The model under review builds one solid part; all positions refer to its coordinate system, in mm. Face numbers are marked on the shaded views. A direction names the side the tool comes from. Coordinates: 2 decimals unless noted, no trailing zeros. Order: outer loops, then holes, each group sorted by start corner. A loop starts at its lowest first (then second) coordinate and runs counter-clockwise, first axis right, second up.
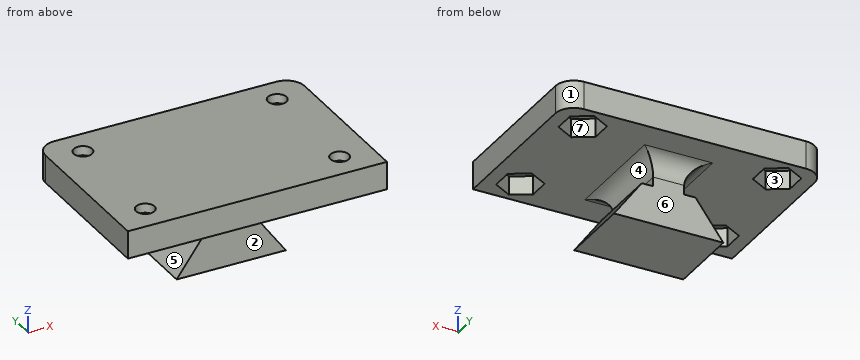
```python
from build123d import *

# Parameters (mm, degrees)
DOVETAIL_DEPTH     = 8
SKETCH2_W          = 3.35034124
SKETCH2_H          = 8
STEM_DEPTH         = 3
SKETCH3_W          = 28
SKETCH3_H          = 18.5
CAMERA_PLATE_DEPTH = 3
FILLET1_R          = 2
SKETCH4_R          = 1
SCREW_HOLES_DEPTH  = 3
NUT_HOLES_DEPTH    = 2
FILLET2_R          = 2


with BuildPart() as part:
    # Sketch1 → Dovetail (new body)
    with BuildSketch(Plane(origin=(0, 0, 0), x_dir=(1, 0, 0), z_dir=(0, 1, 0))):
        Polygon((-2.9, 0), (-5.9, 4.129145761), (5.9, 4.129145761), (2.9, 0), align=None)
    extrude(amount=DOVETAIL_DEPTH)

    # Sketch2 → Stem (add)
    with BuildSketch(Plane.XY):
        with Locations((0, 4)):
            Rectangle(SKETCH2_W, SKETCH2_H)
    extrude(amount=STEM_DEPTH)

    # Sketch3 → Camera Plate (add)
    with BuildSketch(Plane.XY.offset(3)):
        with Locations((0, 4)):
            Rectangle(SKETCH3_W, SKETCH3_H)
    extrude(amount=CAMERA_PLATE_DEPTH)

    # Fillet1
    fillet1_edges = [part.edges().sort_by_distance(p)[0] for p in [
        (1.67517062, 4, 3),
        (0, 8, 3),
        (-1.67517062, 4, 3),
        (0, 0, 3),
    ]]
    fillet(fillet1_edges, radius=FILLET1_R)

    # Sketch4 → Screw Holes (cut)
    with BuildSketch(Plane.XY.offset(6)):
        with Locations((-10.5, 10.25)):
            Circle(SKETCH4_R)
        with Locations((10.5, 10.25)):
            Circle(SKETCH4_R)
        with Locations((10.5, -2.25)):
            Circle(SKETCH4_R)
        with Locations((-10.5, -2.25)):
            Circle(SKETCH4_R)
    extrude(amount=-SCREW_HOLES_DEPTH, mode=Mode.SUBTRACT)

    # Sketch5 → Nut Holes (cut)
    with BuildSketch(Plane(origin=(0, 0, 3), x_dir=(-1, 0, 0), z_dir=(0, 0, -1))):
        Polygon((-10.5, 12.559401077), (-12.5, 11.404700538), (-12.5, 9.095299462), (-10.5, 7.940598923), (-8.5, 9.095299462), (-8.5, 11.404700538), align=None)
        Polygon((10.5, 12.559401077), (8.5, 11.404700538), (8.5, 9.095299462), (10.5, 7.940598923), (12.5, 9.095299462), (12.5, 11.404700538), align=None)
        Polygon((-10.5, -4.559401077), (-8.5, -3.404700538), (-8.5, -1.095299462), (-10.5, 0.059401077), (-12.5, -1.095299462), (-12.5, -3.404700538), align=None)
        Polygon((10.5, -4.559401077), (12.5, -3.404700538), (12.5, -1.095299462), (10.5, 0.059401077), (8.5, -1.095299462), (8.5, -3.404700538), align=None)
    extrude(amount=-NUT_HOLES_DEPTH, mode=Mode.SUBTRACT)

    # Fillet2
    fillet2_edges = [part.edges().sort_by_distance(p)[0] for p in [
        (14, 13.25, 4.5),
        (-14, 13.25, 4.5),
    ]]
    fillet(fillet2_edges, radius=FILLET2_R)


solid = part.part
```
(1) We need section A-A, the plane x = -2.5. Write out the cut boundary in (y, z).
A:
outline: (-5.25, 3) - (-2, 3) arc R2 cw to (-0.82, 2.62) - (8.82, 2.62) arc R2 cw to (10, 3) - (13.25, 3) - (13.25, 6) - (-5.25, 6) - close; (0, -4.13) - (8, -4.13) - (8, 0) - (0, 0) - close
(2) Wall thickness on probe 1 along Y at (x, z) = (-10.5, 5.25); probe 2 along Z at (x, y) = (-7.25, 1.25); probe 3 along Z at (x, y) = (2.25, 4.25): over which ranges is each line inside the solid? List them lowest first.
A:
probe 1: y = -5.25 to -3.25, -1.25 to 9.25, 11.25 to 13.25
probe 2: z = 3 to 6
probe 3: z = -4.13 to 0, 2.4 to 6
(3) Draft analysis for pull direction Y (two halves, no side actions). For the marked faces 5, 6 and 7, state which applies: released by +Y, released by -Y, zero draft, split by the parting line, or undercut.
A:
face 5: zero draft
face 6: released by +Y
face 7: undercut
(4) Machinability: for the marked faces 1, 2, 3 and 4, which of the approach directions +Z, -Z, +X, -X, +Y, -Y give a long, thin tool a straight path to every point of the face, cutting with its end or side? Answer none if there is none.
A:
face 1: +Z, -Z, +X, +Y
face 2: -Z, +X, -X, -Y
face 3: -Z
face 4: +X, +Y, -Y
(5) We need section C-C, the plane z = 2.5. Write out the cut boundary in (x, y), and give its area (3 significant figures).
A:
outline: (-2.35, -0.68) - (2.35, -0.68) - (2.35, 8.68) - (-2.35, 8.68) - close
area: 44.0 mm2
(6) We need section D-D, the plane x = -7.25. Write out the cut boundary in (y, z), and give its area (3 significant figures).
A:
outline: (-5.25, 3) - (13.25, 3) - (13.25, 6) - (-5.25, 6) - close
area: 55.5 mm2
(7) For pin 1 Ø4 at (x, z) = (0.5, -2) entering from -Y; pin 2 Ø4 at (y, z) = (2.5, 0) entering from +X; pin 3 Ø4.5 at (x, y) = (11, -1) entering from -Z; pin 4 Ø1 at (y, z) = (-1, 0.5) entering from +X, all flat-tipped, find the tip position at first contact; note any pin that passes through.
A:
pin 1: stops at y = 0
pin 2: stops at x = 4.35
pin 3: stops at z = 3
pin 4: passes through
(8) We need section B-B, the plane y = 4.5. Write out the cut boundary in (x, z), and give its area (3 significant figures).
A:
outline: (-14, 3) - (-3.68, 3) arc R2 cw to (-1.68, 1) - (-1.68, 0) - (-2.9, 0) - (-5.9, -4.13) - (5.9, -4.13) - (2.9, 0) - (1.68, 0) - (1.68, 1) arc R2 cw to (3.68, 3) - (14, 3) - (14, 6) - (-14, 6) - close
area: 132 mm2
